Check sheet for the modelled part. Datum: model origin and axes. Units: mm. A direction names the side the tool comes from. Coordinates: 2 decimals unless noted, no trailing zeros. Loops run counter-clockwise (first coordinate to the right, second up) from the corner with the lowest first, then second, coordinate; pieces in that order, holes last. Notation, with made-up numbers: (45, 15.25) - (60, 15.25) arc R19 ccw to (60, 22.25) - close; hole circle Ø1 at (-0.5, 75). An arc over 180 degrees is marked (long way). Answer as a JSON object with one key per item and string values. Group by question number.
from build123d import *

# Parameters (mm, degrees)
SKETCH2_R                            = 2
SKETCH2_R_2                          = 1.999999996
MAIN_FLOOR_EXTRUDE_DEPTH             = 5
MAIN_FLOOR_CHAMFER_SIZE              = 1
MOUNT_SCREW_COUNTERSINK_DEPTH        = 3
MOUNT_SCREW_COUNTERSINK_CHAMFER_SIZE = 1


with BuildPart() as part:
    # Sketch2 → Main Floor Extrude (new body)
    with BuildSketch(Plane(origin=(0, 0, 0), x_dir=(1, 0, 0), z_dir=(0, 1, 0))):
        Polygon((129.222330464, 0), (129.222330464, -24.28090912), (82.337763357, -71.165476227), (89.511362957, -78.339075827), (91.560037368, -85.984832777), (85.984832777, -91.560037368), (78.339075822, -89.511362977), (71.165476214, -82.33776337), (24.280909108, -129.222330477), (0, -129.222330477), (-24.28090912, -129.222330477), (-71.165476227, -82.33776337), (-78.339075827, -89.51136297), (-85.984832777, -91.560037381), (-91.560037368, -85.984832789), (-89.511362977, -78.339075834), (-82.33776337, -71.165476227), (-129.222330477, -24.28090912), (-129.222330477, -1.3e-08), (-129.222330477, 24.280909108), (-82.33776337, 71.165476214), (-89.51136297, 78.339075814), (-91.560037381, 85.984832764), (-85.984832789, 91.560037355), (-78.339075834, 89.511362964), (-71.165476227, 82.337763357), (-24.28090912, 129.222330464), (-1.3e-08, 129.222330464), (24.280909108, 129.222330464), (71.165476214, 82.337763357), (78.339075814, 89.511362957), (85.984832764, 91.560037368), (91.560037355, 85.984832777), (89.511362964, 78.339075822), (82.337763357, 71.165476214), (129.222330464, 24.280909108), align=None)
        with Locations(Location((86.014718626, -86.014718626, 0), (0, 0, 270))):
            Circle(SKETCH2_R, mode=Mode.SUBTRACT)
        with Locations(Location((-86.014718626, -86.014718639, 0), (0, 0, 270))):
            Circle(SKETCH2_R, mode=Mode.SUBTRACT)
        with Locations(Location((-86.014718639, 86.014718613, 0), (0, 0, 270))):
            Circle(SKETCH2_R, mode=Mode.SUBTRACT)
        with Locations(Location((86.014718613, 86.014718626, 0), (0, 0, 270))):
            Circle(SKETCH2_R_2, mode=Mode.SUBTRACT)
    extrude(amount=MAIN_FLOOR_EXTRUDE_DEPTH)

    # Main Floor Chamfer
    main_floor_chamfer_edges = [part.edges().sort_by_distance(p)[0] for p in [
        (-74.752276027, 5, 85.92456317),
        (-47.723192674, 5, 105.780046923),
        (-6e-09, 5, 129.222330477),
        (47.723192661, 5, 105.780046923),
        (74.752276018, 5, 85.924563174),
        (82.161954299, 5, 90.535700173),
        (88.772435072, 5, 88.772435072),
        (85.924563161, 5, -74.752276018),
        (90.535700163, 5, 82.161954302),
        (85.924563157, 5, 74.752276027),
        (105.780046911, 5, 47.723192674),
        (90.53570016, 5, -82.161954299),
        (88.77243506, 5, -88.772435072),
        (82.161954289, 5, -90.535700163),
        (74.752276014, 5, -85.924563157),
        (47.723192661, 5, -105.780046911),
        (-6e-09, 5, -129.222330464),
        (-47.723192674, 5, -105.780046911),
        (-74.752276031, 5, -85.924563161),
        (129.222330464, 5, 6e-09),
        (-82.161954312, 5, -90.53570016),
        (-88.772435085, 5, -88.77243506),
        (-90.535700175, 5, -82.161954289),
        (-85.92456317, 5, -74.752276014),
        (-105.780046923, 5, -47.723192661),
        (-129.222330477, 5, 6e-09),
        (-105.780046923, 5, 47.723192674),
        (-85.924563174, 5, 74.752276031),
        (-90.535700173, 5, 82.161954312),
        (105.780046911, 5, -47.723192661),
        (-88.772435072, 5, 88.772435085),
        (-82.161954302, 5, 90.535700175),
    ]]
    chamfer(main_floor_chamfer_edges, length=MAIN_FLOOR_CHAMFER_SIZE)

    # Sketch3 → Mount Screw Countersink (cut)
    with BuildSketch(Plane(origin=(0, 0, 0), x_dir=(-1, 0, 0), z_dir=(0, -1, 0))):
        with BuildLine():
            Line((91.247308807, -86.297561351), (88.48959236, -83.539844904))
            ThreePointArc((88.48959236, -83.539844904), (83.539844892, -83.539844904), (83.539844892, -88.489592373))
            Line((83.539844892, -88.489592373), (86.297561338, -91.247308819))
            Line((86.297561338, -91.247308819), (91.247308807, -86.297561351))
        make_face()
        with BuildLine():
            Line((-86.297561351, -91.247308807), (-83.539844904, -88.48959236))
            ThreePointArc((-83.539844904, -88.48959236), (-83.539844904, -83.539844892), (-88.489592373, -83.539844892))
            Line((-88.489592373, -83.539844892), (-91.247308819, -86.297561338))
            Line((-91.247308819, -86.297561338), (-86.297561351, -91.247308807))
        make_face()
        with BuildLine():
            Line((-91.247308807, 86.297561351), (-88.48959236, 83.539844904))
            ThreePointArc((-88.48959236, 83.539844904), (-83.539844892, 83.539844904), (-83.539844892, 88.489592373))
            Line((-83.539844892, 88.489592373), (-86.297561338, 91.247308819))
            Line((-86.297561338, 91.247308819), (-91.247308807, 86.297561351))
        make_face()
        with BuildLine():
            Line((86.297561351, 91.247308807), (83.539844904, 88.48959236))
            ThreePointArc((83.539844904, 88.48959236), (83.539844904, 83.539844892), (88.489592373, 83.539844892))
            Line((88.489592373, 83.539844892), (91.247308819, 86.297561338))
            Line((91.247308819, 86.297561338), (86.297561351, 91.247308807))
        make_face()
    extrude(amount=-MOUNT_SCREW_COUNTERSINK_DEPTH, mode=Mode.SUBTRACT)

    # Mount Screw Countersink Chamfer
    mount_screw_countersink_chamfer_edges = [part.edges().sort_by_distance(p)[0] for p in [
        (-84.918703128, 0, -89.868450583),
        (-89.868450596, 0, -84.918703115),
        (-83.539844904, 0, -83.539844892),
        (89.868450583, 0, -84.918703128),
        (84.918703115, 0, -89.868450596),
        (83.539844892, 0, -83.539844904),
        (84.918703128, 0, 89.868450583),
        (89.868450596, 0, 84.918703115),
        (83.539844904, 0, 83.539844892),
        (-89.868450583, 0, 84.918703128),
        (-84.918703115, 0, 89.868450596),
        (-83.539844892, 0, 83.539844904),
    ]]
    chamfer(mount_screw_countersink_chamfer_edges, length=MOUNT_SCREW_COUNTERSINK_CHAMFER_SIZE)


solid = part.part
1. Release check for a two-part mould opening along Z. For faces 1 (the face through (88.45, 4.51, 88.37)), 2 (the face through (-74.812, 4.507, -85.268)), 3 (the face through (-83.49, 1.99, -83.59)) record: released by +Z, released by -Z, zero draft, split by the parting line, or undercut.
2. Gauge pin test, flat ends, axial feed: pin 1 (2 mm diameter, centred on y = 0.5, z = -27, fed in from -X); pin 2 (4.5 mm diameter, centred on x = -85, z = 85, fed in from -Y) (3 decimals); pin 3 (4.5 mm diameter, centred on x = 86.01, z = -86.01, fed in from -Y); pin 4 (2.5 mm diameter, centred on x = -86.01, z = -86.01, fed in from -Y). Record the tip position at first contact, or that the pin passes through.
3. Material ranges on line 1 (X direction, y = 4.55, z = 82.5); line 2 (Z direction, x = -89, y = 1.35); line 3 (X direction, y = 1.8, z = -79), recorded low to high.
4. Access from +Z, -Z, +X, -X, +Y, -Y to the whole of each face (thin tool, end or side, straight path). Record for faces 4 (the face through (87, 3, 88)), 5 (the face through (-74.8, 1.97, -85.97)), 6 (the face through (74.812, 4.507, 85.268)), 7 (the face through (105.452, 1.972, -48.051)), 8 (the face through (-47.395, 1.972, 106.108)).
5. Sectioned sample at A-A on x = -57. Record the cut outline in (y, z), plus the area to 3 significant figures.
6. Sectioned sample at B-B on z = 107.5. Record the cut outline in (x, y).
Answers follow:
{
 "1": {"face 1": "released by +Z", "face 2": "released by -Z", "face 3": "undercut"},
 "2": {"pin 1": "stops at x = -127.5", "pin 2": "stops at y = 0.815", "pin 3": "stops at y = 3", "pin 4": "passes through"},
 "3": {"line 1": "x = -90.06 to -72.11, -70.23 to 70.23, 72.11 to 90.06", "line 2": "z = -84.05 to -77.83, -64.5 to 64.5, 77.83 to 84.05", "line 3": "x = -89.69 to 89.69"},
 "4": {"face 4": "-Y", "face 5": "-Z, +Y, -Y", "face 6": "+Z, +Y", "face 7": "+X, +Y, -Y", "face 8": "+Z, +Y, -Y"},
 "5": {"outline": "(0, -96.5) - (4, -96.5) - (5, -95.09) - (5, 95.09) - (4, 96.5) - (0, 96.5) - close", "area": "964 mm^2"},
 "6": {"outline": "(-46, 0) - (46, 0) - (46, 4) - (44.59, 5) - (-44.59, 5) - (-46, 4) - close"}
}
